Source: three-view drawing plus pictorial views. Frame: mm from the lowest corner of the part. Give positions to 0.01 mm unless a question says otherwise; leave off trailing zeros. Order: outer loops, then holes, each group sorted by start corner. A loop starts at its lowest first (then second) coordinate and runs counter-clockwise, first axis right, second up. Notation, with made-up numbers: (-37, 23.5) -> (-22, 23.5) arc R23 ccw to (-22, 48.5) -> close; hole circle Ø6 at (-22.5, 89). An arc over 180 degrees is marked (long way). Write item = value, one per line.
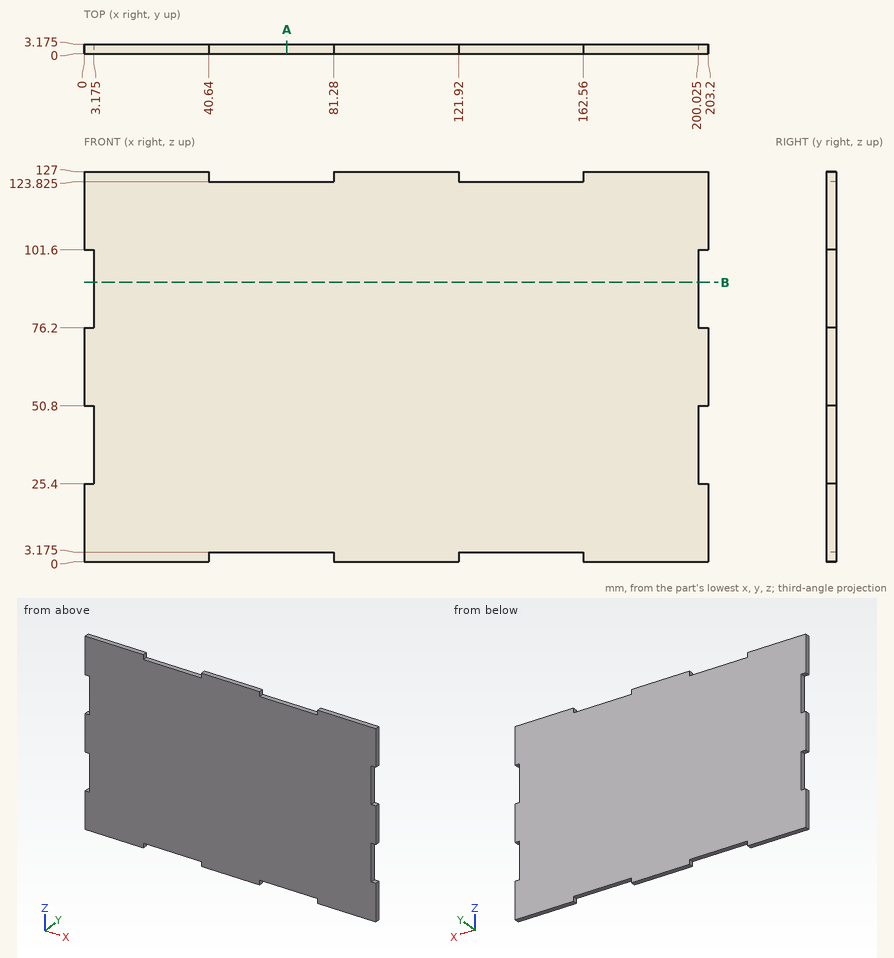
1) Section query A-A (x = 66). Output: boundary loops of the cut face in (y, z) (3 decimals).
Check sheet entries:
outline = (0, 3.175) -> (3.175, 3.175) -> (3.175, 123.825) -> (0, 123.825) -> close
2) Line query: line 1 (X direction, y = 1.55, z = 48.5) (3 decimals); line 2 (Z direction, x = 43.5, y = 2.35) (3 decimals). Output: solid intervals per line, ascending. Write a range as from..to.
Check sheet entries:
line_1 = 3.175..200.025
line_2 = 3.175..123.825
3) Section query B-B (z = 91). Output: boundary loops of the cut face in (x, y) (3 decimals), plus the area to 3 significant figures.
Check sheet entries:
outline = (3.175, 0) -> (200.025, 0) -> (200.025, 3.175) -> (3.175, 3.175) -> close
area = 625 mm²
4) First-contact query: P1, Ø1.5, axis at y = 2, z = 49.5, coming from the +X side (3 decimals); P2, Ø1.6, axis at x = 1, y = 1, coming from the -Z side. Flat tips, straight axial feed; report the tip coordinate or a pass-through.
Check sheet entries:
P1 = 200.025
P2 = 0
